Source: CAD feature listing. Evaluate the final solid. Frame: model axes, mm. A direction names the side the tool comes from. Coordinates: 2 decimals unless noted, no trailing zeros. Write each loop counter-clockwise with the first axis right and the second up, starting at its lowest first coordinate (ties: lowest second). Pieces come first, ordered by that corner, then holes. Notation, with made-up numbers: (-1, 64.25) - (32, 64.25) arc R16 ccw to (32, 70.25) - close; hole circle Ø7 at (68, 85). An arc over 180 degrees is marked (long way). One line per question, with ' | ' between items. Start each with the question number.
Q1. Cut plane A-A, the plane z = -28. Return loops of the section in (x, y), plus the area to 3 significant figures.
Q2. Cut plane B-B, the plane y = -12. Return loops of the section in (x, z).
Q3. Line query: line 1 (Y direction, x = -17.5, z = 28); line 2 (Z direction, x = -5.75, y = -12); line 3 (Z direction, x = -21.75, y = -12). Output: solid intervals per line, ascending.
Q4. Access query for faces 1 (the face through (-25, -12, 24)), 2 (the face through (-25, -12, -24)), 3 (the face through (-19, -12, 23)), 4 (the face through (-26, -12, 22)), 5 (the face through (-32, -17, 5)). Directions: +Z, -Z, +X, -X, +Y, -Y. A direction counts if a zero-diameter tool reaches every point of the face in a straight line with its end or side. Return the directions, or none.
Q5. Cut plane C-C, the plane x = -10. Return loops of the section in (y, z).
Q6. Draft query along X for faces 6 (the face through (-22, -25, 0)), 7 (the face through (0, -15, 27)), 8 (the face through (-15, -14, -25)). Return one class per face: +X half, -X half, draft (parallel to the pull), parting line (faces both ways), or undercut.
Q7. Cut plane D-D, the plane y = -23. Return loops of the section in (x, z), plus the area to 3 significant figures.
Q8. Contact query for flat-ended pins moving along their axis: P1, Ø5.5, axis at x = -33, z = 8, coming from the -Y side; P2, Ø4, axis at y = -17.5, z = -16, coming from the -X side; P3, Ø4.5, axis at y = -10.5, z = 27, coming from the -X side. Output: stop coordinate, or through.
```python
from build123d import *

# Parameters (mm, degrees)
F1_DEPTH  = 25
F2_R      = 3
F3_DEPTH  = 25
F5_R      = 5
F6_DEPTH  = 5
F8_DEPTH  = 28.5
F9_W      = 8
F9_H      = 14
F10_DEPTH = 25


with BuildPart() as f1:
    # F0 (on Front) → F1 (new body)
    with BuildSketch(Plane.XZ):
        with BuildLine():
            Line((0, 20), (0, 35))
            ThreePointArc((0, 35), (-35, 0), (0, -35))
            Line((0, -35), (0, -20))
            ThreePointArc((0, -20), (-20, 0), (0, 20))
        make_face()
    extrude(amount=F1_DEPTH)

    # F2 (on Right) → F3 (cut)
    with BuildSketch(Plane.YZ):
        with Locations((-12, 28)):
            Circle(F2_R)
        with Locations((-12, -28)):
            Circle(F2_R)
    extrude(amount=-F3_DEPTH, mode=Mode.SUBTRACT)

    # F5 (on offset) → F6 (cut, symmetric)
    with BuildSketch(Plane.YZ.offset(-20)):
        with Locations((-12, 28)):
            Circle(F5_R)
        with Locations((-12, -28)):
            Circle(F5_R)
    extrude(amount=F6_DEPTH, both=True, mode=Mode.SUBTRACT)

    # F7 (on Front) → F8 (cut)
    with BuildSketch(Plane.XZ):
        Polygon((-30, 0), (-24, 0), (-24, 14), (-24, 22), (-30, 22), (-44, 22), (-44, 14), (-30, 14), align=None)
    extrude(amount=F8_DEPTH, mode=Mode.SUBTRACT)

    # F9 (on face) → F10 (cut)
    with BuildSketch(Plane(origin=(-24, 0, 0), x_dir=(0, -1, 0), z_dir=(-1, 0, 0))):
        with Locations((4, 7)):
            Rectangle(F9_W, F9_H)
        with Locations((21, 7)):
            Rectangle(F9_W, F9_H)
    extrude(amount=F10_DEPTH, mode=Mode.SUBTRACT)


solid = f1.part
```
Reply:
1) outline: (-21, -25) - (0, -25) - (0, -15) - (-15, -15) - (-15, -17) - (-21, -17) - close; (-21, -7) - (-15, -7) - (-15, -9) - (0, -9) - (0, 0) - (-21, 0) - close | area: 375 mm^2
2) outline: (-32.08, 14) arc R35 ccw to (-25, -24.49) - (-25, -23) - (-15, -23) - (-15, -25) - (0, -25) - (0, -20) arc R20 cw to (0, 20) - (0, 25) - (-15, 25) - (-15, 23) - (-25, 23) - (-25, 24.49) arc R35 ccw to (-27.22, 22) - (-24, 22) - (-24, 0) - (-30, 0) - (-30, 14) - close; (-15, -31.62) arc R35 ccw to (0, -35) - (0, -31) - (-15, -31) - close; (-15, 31) - (0, 31) - (0, 35) arc R35 ccw to (-15, 31.62) - close
3) line 1: y = -25 to -17, -7 to 0 | line 2: z = -34.52 to -31, -25 to -19.16, 19.16 to 25, 31 to 34.52 | line 3: z = -23 to 23
4) face 1: +Z | face 2: -Z | face 3: none | face 4: -X, +Y, -Y | face 5: +Z, -X, -Y
5) outline: (-25, -33.54) - (0, -33.54) - (0, -17.32) - (-25, -17.32) - close; (-25, 17.32) - (0, 17.32) - (0, 33.54) - (-25, 33.54) - close; hole circle Ø6 at (-12, -28); hole circle Ø6 at (-12, 28)
6) face 6: draft | face 7: +X half | face 8: undercut
7) outline: (-35, 0) arc R35 ccw to (0, -35) - (0, -20) arc R20 cw to (0, 20) - (0, 35) arc R35 ccw to (-27.22, 22) - (-24, 22) - (-24, 0) - close | area: 1,110 mm^2
8) P1: stops at y = -17 | P2: stops at x = -32.08 | P3: stops at x = -15
